Read the model definition and answer for the solid it produces. Units are mm, in the model's axes. A direction names the side the tool comes from. Give positions to 0.01 mm unless a question says otherwise; leave off trailing zeros. Order: outer loops, then holes, each group sorted by start corner. A loop starts at its lowest first (then second) coordinate and runs counter-clockwise, first axis right, second up. Notation, with made-up numbers: (-18, -6) - (-10, -6) arc R24 ccw to (-10, 30) - close; hole circle Ø8 at (-40, 30). An arc over 180 degrees is marked (long way). Use a Markdown table: item, result. Add a question column.
1. Consider L1, parallel to X at y = -2, z = 5.5; L2, parallel to Z at x = 12, y = -3.5; L3, parallel to X at y = -4.75, z = 24.75. Determine where each line is inside the solid, lowest interval first.
2. Which of the six approach directions +Z, -Z, +X, -X, +Y, -Y give full straight-line access (tool end or side, diameter ignored) to faces 1 (the flat face through (21, -3, 6.874)), 2 (the flat face through (16, 0, 11))?
3. For a pull along X with two mould halves and no side action, classify faces 3 (the flat face through (16, -6.35, 11)), 4 (the flat face through (12.7, -3, 5)), 5 (the flat face through (8.05, -3.13, 20.72)) as released by +X, released by -X, zero draft, split by the parting line, or undercut.
4. Flat-ended cylindrical pins translate along their axes: P1, Ø1.4, axis at x = 20.5, y = -4, coming from the +Z side; P2, Ø2, axis at x = 19, y = -1.5, coming from the +Z side; P3, Ø1, axis at y = -3.5, z = 22.5, coming from the +X side. Find the tip coordinate at first contact, or state that the pin passes through.
5. A cutting plane is placed at C-C on y = -2.75. State how many separate pieces and enclosed holes the cut face has, and give its area (3 significant figures).
6. A cutting plane is placed at A-A on x = 10. Determine the outline of the cut face in (y, z).
7. A cutting plane is placed at B-B on z = 15.5. Determine the outline of the cut face in (x, y).
8. A cutting plane is placed at D-D on z = 24.5. Determine the outline of the cut face in (x, y).
```python
from build123d import *

# Parameters (mm, degrees)
F1_DEPTH = 6.35


# Not quite as in the source:
# - a feature names something its author has since deleted; it is built from what else it names


with BuildPart() as f1:
    # F0 (on Front) → F1 (new body)
    with BuildSketch(Plane.XZ):
        Polygon((1.984375, 3.4370383213), (0, 0), (7.9375, 0), (15.875, 0), (31.75, 0), (29.765625, 3.4370383213), (23.8125, 3.4370383213), (19.05, 3.4370383213), (15.875, 3.4370383213), (12.7, 3.4370383213), (11.90625, 3.4370383213), (7.9375, 3.4370383213), align=None)
        Polygon((0, 3.4370383213), (0, 0), (1.984375, 3.4370383213), align=None)
        Polygon((0, 3.4370383213), (1.984375, 3.4370383213), (7.9375, 13.7481532851), (0, 13.7481532851), (0, 6.8740766425), align=None)
        with BuildLine():
            Line((7.9375, 13.7481532851), (1.984375, 3.4370383213))
            Line((1.984375, 3.4370383213), (7.9375, 3.4370383213))
            Line((7.9375, 3.4370383213), (7.9375, 6.8740766425))
            Line((7.9375, 6.8740766425), (12.7, 6.8740766425))
            Line((12.7, 6.8740766425), (15.875, 6.8740766425))
            Line((15.875, 6.8740766425), (19.05, 6.8740766425))
            Line((19.05, 6.8740766425), (23.8125, 6.8740766425))
            Line((23.8125, 6.8740766425), (23.8125, 3.4370383213))
            Line((23.8125, 3.4370383213), (29.765625, 3.4370383213))
            Line((29.765625, 3.4370383213), (23.8125, 13.7481532851))
            Line((23.8125, 13.7481532851), (19.1716913456, 13.7481532851))
            ThreePointArc((19.1716913456, 13.7481532851), (15.875, 12.4226916063), (12.5783086544, 13.7481532851))
            Line((12.5783086544, 13.7481532851), (7.9375, 13.7481532851))
        make_face()
        Polygon((0, 13.7481532851), (7.9375, 13.7481532851), (15.875, 27.4963065702), align=None)
        with BuildLine():
            Line((15.875, 27.4963065702), (7.9375, 13.7481532851))
            Line((7.9375, 13.7481532851), (12.5783086544, 13.7481532851))
            ThreePointArc((12.5783086544, 13.7481532851), (14.0067235595, 21.56593919), (20.6375, 17.1851916063))
            ThreePointArc((20.6375, 17.1851916063), (20.2557475837, 15.3169151658), (19.1716913456, 13.7481532851))
            Line((19.1716913456, 13.7481532851), (23.8125, 13.7481532851))
            Line((23.8125, 13.7481532851), (15.875, 27.4963065702))
        make_face()
        Polygon((29.765625, 3.4370383213), (31.75, 0), (31.75, 3.4370383213), align=None)
        Polygon((31.75, 13.7481532851), (15.875, 27.4963065702), (23.8125, 13.7481532851), align=None)
        Polygon((23.8125, 13.7481532851), (29.765625, 3.4370383213), (31.75, 3.4370383213), (31.75, 13.7481532851), align=None)
        Polygon((12.7, 6.8740766425), (12.7, 3.4370383213), (15.875, 3.4370383213), (19.05, 3.4370383213), (19.05, 6.8740766425), (15.875, 6.8740766425), align=None)
    extrude(amount=F1_DEPTH)


solid = f1.part
```
Output values:
| question | item | result |
|---|---|---|
| 1 | L1 | 0 to 7.94, 12.7 to 19.05, 23.81 to 31.75 |
| 1 | L2 | 0 to 3.44, 6.87 to 14.42, 19.95 to 24.14 |
| 1 | L3 | 12.7 to 19.05 |
| 2 | face 1 | +Y, -Y |
| 2 | face 2 | +Z, -Z, +X, -X, +Y |
| 3 | face 3 | zero draft |
| 3 | face 4 | undercut |
| 3 | face 5 | released by -X |
| 4 | P1 | z = 24.1 |
| 4 | P2 | z = 25.66 |
| 4 | P3 | x = 22.22 |
| 5 | separate pieces | 1 |
| 5 | enclosed holes | 3 |
| 5 | area | 551 mm² |
| 6 | outline | (-6.35, 0) - (0, 0) - (0, 3.44) - (-6.35, 3.44) - close; (-6.35, 6.87) - (0, 6.87) - (0, 22.41) - (-6.35, 22.41) - close |
| 7 | outline | (2.02, -6.35) - (11.42, -6.35) - (11.42, 0) - (2.02, 0) - close; (20.33, -6.35) - (29.73, -6.35) - (29.73, 0) - (20.33, 0) - close |
| 8 | outline | (12.42, -6.35) - (19.33, -6.35) - (19.33, 0) - (12.42, 0) - close |
